```python
from build123d import *

# Parameters (mm, degrees)
BOSS_EXTRUDE1_DEPTH      = 20
SKETCH2_R                = 5.1
SKETCH2_R_2              = 1.75
CUT_EXTRUDE1_DEPTH       = 98.821265582
CUT_EXTRUDE2_DEPTH       = 109.023145668
F_4_0_4_DIAMETER_HOLE1_D = 4


with BuildPart() as part:
    # Sketch1 → Boss-Extrude1 (new, symmetric)
    with BuildSketch(Plane.XY):
        Polygon((0, 0), (0, 87), (-50, 87), (-50, 77), (-10, 77), (-10, 0), align=None)
    extrude(amount=BOSS_EXTRUDE1_DEPTH, both=True)

    # Sketch2 → Cut-Extrude1 (cut, through all)
    with BuildSketch(Plane.ZY.offset(10)):
        with Locations(Location((0, 11, 0), (0, 0, 270))):
            Circle(SKETCH2_R)
        with Locations(Location((5.656854249, 16.656854249, 0), (0, 0, 270))):
            Circle(SKETCH2_R_2)
        with Locations(Location((5.656854249, 5.343145751, 0), (0, 0, 270))):
            Circle(SKETCH2_R_2)
        with Locations(Location((-5.656854249, 16.656854249, 0), (0, 0, 270))):
            Circle(SKETCH2_R_2)
        with Locations(Location((-5.656854249, 5.343145751, 0), (0, 0, 270))):
            Circle(SKETCH2_R_2)
    extrude(amount=-CUT_EXTRUDE1_DEPTH, mode=Mode.SUBTRACT)

    # Sketch3 → Cut-Extrude2 (cut, through all)
    with BuildSketch(Plane.XY.offset(20)):
        Polygon((0, 0), (-10, 0), (-10, 30), (-5, 30), (-5, 40), (0, 40), align=None)
    extrude(amount=-CUT_EXTRUDE2_DEPTH, mode=Mode.SUBTRACT)

    # Ø4.0 (4) Diameter Hole1 (through all)
    with Locations(Plane(origin=(-5, 0, 0), x_dir=(0, 0, -1), z_dir=(1, 0, 0))):
        with Locations((-12.5, 35), (0, 35), (12.5, 35)):
            Hole(F_4_0_4_DIAMETER_HOLE1_D / 2)


solid = part.part
```
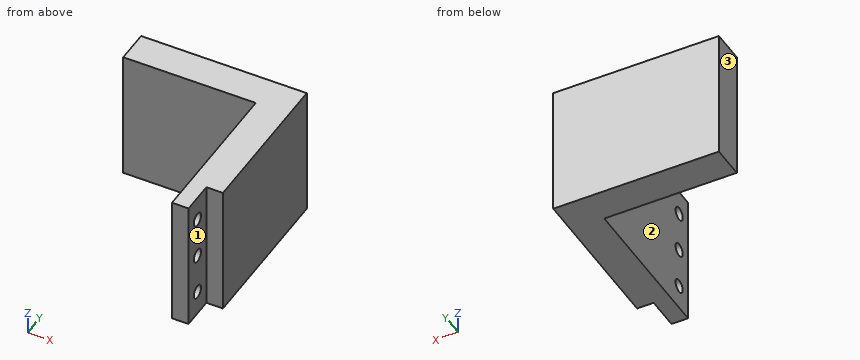
Model file for the job. Use its own axes, mm. Face numbers are marked on the shaded views. A direction names the side the tool comes from. Coordinates: 2 decimals unless noted, no trailing zeros. Order: outer loops, then holes, each group sorted by start corner. A loop starts at its lowest first (then second) coordinate and runs counter-clockwise, first axis right, second up. Notation, with made-up numbers: M 81.25,83.25 L 137.25,83.25 A26 cw 137.25,109.25 Z; hole C 5.25,-21 d7. An arc over 180 degrees is marked long. Answer as CSV lines item,"result".
(1) Wall check: line 1 along Y through (x, z) = (-7.1, 0); line 2 along X through (y, z) = (52, 2); line 3 along Y through (x, z) = (-46, -5). Give the ranges that are in metal, low to high.
Geometry says:
line 1,"y = 30 to 33, 37 to 87"
line 2,"x = -10 to 0"
line 3,"y = 77 to 87"
(2) 3-axis set-ups, long thin cutter, end or side, ignore diameter. For the marked faces 1, 2 and 3: which of +Z, -Z, +X, -X, +Y, -Y reach the whole face in a straight line?
Geometry says:
face 1,"+Z, -Z, +X, -Y"
face 2,"+Z, -Z, -X, -Y"
face 3,"+Z, -Z, -X, +Y, -Y"
(3) Band-saw the part on D-D, the plane x = -20. List the corners of the cut face in (y, z), then the cut area to 3 significant figures.
Geometry says:
outline,"M 77,-20 L 87,-20 L 87,20 L 77,20 Z"
area,"400 mm2"
(4) Band-saw the part on A-A, the plane y = 35. List the corners of the cut face in (x, z), then the cut area to 3 significant figures.
Geometry says:
outline,"M -10,-20 L -5,-20 L -5,-14.5 L -10,-14.5 Z; M -10,-10.5 L -5,-10.5 L -5,-2 L -10,-2 Z; M -10,2 L -5,2 L -5,10.5 L -10,10.5 Z; M -10,14.5 L -5,14.5 L -5,20 L -10,20 Z"
area,"140 mm2"
(5) Flat gauge pins, fed straight in: pin 1 (3 mm diameter, centred on y = 36, z = 9, fed in from +X); pin 2 (3 mm diameter, centred on y = 35, z = 12.5, fed in from -X); pin 3 (6.5 mm diameter, centred on y = 35, z = -12.5, fed in from -X); pin 4 (3 mm diameter, centred on x = -18, z = 13, fed in from -Y). Where does each tip first touch, or does it go through?
Geometry says:
pin 1,"stops at x = -5"
pin 2,"passes through"
pin 3,"stops at x = -10"
pin 4,"stops at y = 77"
(6) Band-saw the part on C-C, the plane z = -5. List the corners of the cut face in (x, y), then the cut area to 3 significant figures.
Geometry says:
outline,"M -50,77 L -10,77 L -10,30 L -5,30 L -5,40 L 0,40 L 0,87 L -50,87 Z"
area,"920 mm2"
(7) Band-saw the part on B-B, the plane z = 0. List the corners of the cut face in (x, y), then the cut area to 3 significant figures.
Geometry says:
outline,"M -50,77 L -10,77 L -10,37 L -5,37 L -5,40 L 0,40 L 0,87 L -50,87 Z; M -10,30 L -5,30 L -5,33 L -10,33 Z"
area,"900 mm2"
